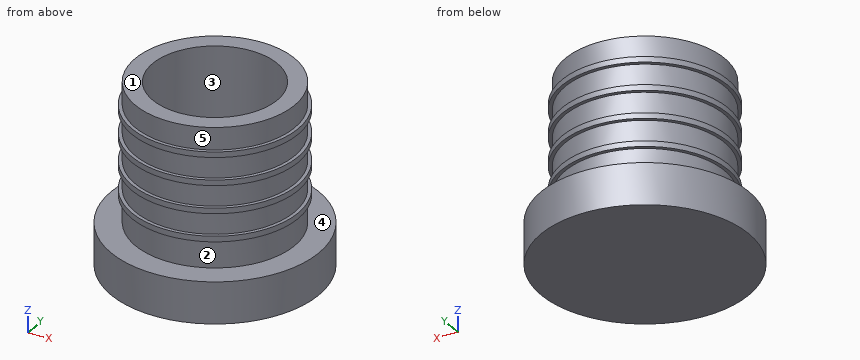
from build123d import *

# Parameters (mm, degrees)
F0_R      = 7.5
F1_DEPTH  = 3
F2_R      = 5.75
F2_R_2    = 4.5
F3_DEPTH  = 10
F5_R      = 6
F5_R_2    = 4.5
F6_DEPTH  = 0.4
F8_R      = 6
F8_R_2    = 4.5
F9_DEPTH  = 0.4
F11_R     = 6
F11_R_2   = 4.5
F12_DEPTH = 0.4
F14_R     = 6
F14_R_2   = 4.5
F15_DEPTH = 0.4


with BuildPart() as f1:
    # F0 (on Top) → F1 (new body)
    with BuildSketch(Plane.XY):
        Circle(F0_R)
    extrude(amount=F1_DEPTH)

    # F2 (on face) → F3 (join)
    with BuildSketch(Plane.XY.offset(3)):
        Circle(F2_R)
        Circle(F2_R_2, mode=Mode.SUBTRACT)
    extrude(amount=F3_DEPTH)

    # F5 (on offset) → F6 (join)
    with BuildSketch(Plane.XY.offset(5)):
        Circle(F5_R)
        Circle(F5_R_2, mode=Mode.SUBTRACT)
    extrude(amount=F6_DEPTH)

    # F8 (on offset) → F9 (join)
    with BuildSketch(Plane.XY.offset(7)):
        Circle(F8_R)
        Circle(F8_R_2, mode=Mode.SUBTRACT)
    extrude(amount=F9_DEPTH)

    # F11 (on offset) → F12 (join)
    with BuildSketch(Plane.XY.offset(9)):
        Circle(F11_R)
        Circle(F11_R_2, mode=Mode.SUBTRACT)
    extrude(amount=F12_DEPTH)

    # F14 (on offset) → F15 (join)
    with BuildSketch(Plane.XY.offset(11)):
        Circle(F14_R)
        Circle(F14_R_2, mode=Mode.SUBTRACT)
    extrude(amount=F15_DEPTH)


solid = f1.part
The listing builds one solid part. Answer for the finished solid, in the listing's coordinates (mm). Face numbers are marked on the shaded views. A direction names the side the tool comes from. Coordinates: 2 decimals unless noted, no trailing zeros. Loops run counter-clockwise (first coordinate to the right, second up) from the corner with the lowest first, then second, coordinate; pieces in that order, holes last. Notation, with made-up numbers: (-0.5, 32) -> (44.5, 32) arc R15 cw to (44.5, 50) -> close; hole circle Ø5 at (57, 25). An arc over 180 degrees is marked (long way). Answer in a Markdown table with one row per item. Add a question column.
1. The part is cut by section A-A, the plane z = 4. Write down the section's boundary in (x, y), then the cut area to 3 significant figures.
2. For the marked faces 1 and 2, determine the directions among +Z, -Z, +X, -X, +Y, -Y from which every point of the face is accessible in a straight line to the end or side of a thin tool.
3. Flat-ended cylindrical pins translate along their axes: P1, Ø3, axis at y = -1.5, z = 8.5, coming from the +X side; P2, Ø6, axis at x = -1, y = -3, coming from the -Z side; P3, Ø4.5, axis at x = 0, y = 0, coming from the +Z side; P4, Ø1.5, axis at x = 5, z = 11, coming from the +Y side. Find the tip coordinate at first contact, or state that the pin passes through.
4. Determine the mould class of the marked faces 3, 4 and 5 for opening direction Y: +Y half, -Y half, draft (parallel to the pull), parting line (faces both ways), or undercut.
5. Consider line 1 (Y direction, x = 0, z = 6.25); line 2 (Z direction, x = 0, y = 0); line 3 (X direction, y = 3, z = 8.5). Determine where each line is inside the solid, lowest interval first. Write a range as [from, to].
Answer below:
| question | item | result |
|---|---|---|
| 1 | outline | circle Ø11.5 at (0, 0); hole circle Ø9 at (0, 0) |
| 1 | area | 40.3 mm2 |
| 2 | face 1 | +Z, +X, -X, +Y, -Y |
| 2 | face 2 | none |
| 3 | P1 | x = 6 |
| 3 | P2 | z = 0 |
| 3 | P3 | z = 3 |
| 3 | P4 | y = 4.24 |
| 4 | face 3 | undercut |
| 4 | face 4 | draft |
| 4 | face 5 | parting line |
| 5 | line 1 | [-5.75, -4.5], [4.5, 5.75] |
| 5 | line 2 | [0, 3] |
| 5 | line 3 | [-4.91, -3.35], [3.35, 4.91] |
